Part model, mm, in its own coordinate system. A direction names the side the tool comes from. Coordinates: 2 decimals unless noted, no trailing zeros. Loops run counter-clockwise (first coordinate to the right, second up) from the corner with the lowest first, then second, coordinate; pieces in that order, holes last. Notation, with made-up numbers: (9.25, 62) -> (39.25, 62) arc R21 cw to (39.25, 100) -> close; hole circle Ø3 at (53.25, 4). An arc over 180 degrees is marked (long way). Use one line per item in the form item = value. Start each with the question number.
(1) Band-saw the part on C-C on z = 8. Give the cut face in (x, y), then the cut area to 3 significant figures.
(2) Band-saw the part on B-B on z = 38. Give the cut face in (x, y), then the cut area to 3 significant figures.
(3) 3-axis set-ups, long thin cutter, end or side, ignore diameter. For faces 1 (the flat face through (-30.894, -6.088, 0.493)), 2 (the flat face through (-6.35, 8, 6)), 3 (the flat face through (-30.37, -6.08, 24.66)): which of +Z, -Z, +X, -X, +Y, -Y reach the whole face in a straight line?
(4) Pin check, flat tips, straight feed: P1, Ø2, axis at x = -5, z = 21, coming from the -Y side; P2, Ø6, axis at y = 6, z = 42, coming from the +X side; P3, Ø1, axis at y = -5, z = 8, coming from the +X side. Stop position of each tip, or through.
(5) Band-saw the part on D-D on x = -3. Give the cut face in (y, z), then the cut area to 3 significant figures.
(6) Mould opens along Z. For faces 4 (the flat face through (-24, 3, 50)), 5 (the cylindrical face through (-3.131, 5.349, 46.957)), 6 (the flat face through (-34, -12, 25)) say: +Z half, -Z half, draft (parallel to the pull), parting line (faces both ways), or undercut.
(7) Band-saw the part on A-A on y = 6. Give the cut face in (x, z), then the cut area to 3 significant figures.
(8) Drill centre lines: L1, parallel to Z at x = -1.25, y = 6; L2, parallel to Z at x = -16, y = 6; L3, parallel to Y at x = -8, z = 12.5. Where is each one in solid material? Low to high. Write a range as [from, to].
```python
from build123d import *

# Parameters (mm, degrees)
F1_DEPTH       = 50
F3_D           = 5.1054
F3_CBORE_D     = 10
F3_CBORE_DEPTH = 6.35
F4_SIZE        = 1


with BuildPart() as f1:
    # F0 (on Top) → F1 (new body)
    with BuildSketch(Plane.XY):
        Polygon((-32, 0), (0, 0), (0, 12), (-38.78461, 12), (-38.78461, -12), (-28.78461, -12), align=None)
    extrude(amount=F1_DEPTH)

    # F3 (through all)
    with Locations(Plane.YZ):
        with Locations((6, 42), (6, 8)):
            CounterBoreHole(F3_D / 2, F3_CBORE_D / 2, F3_CBORE_DEPTH)

    # F4
    f4_edges = [f1.edges().sort_by_distance(p)[0] for p in [
        (-30.392305, -6, 50),
        (-30.392305, -6, 0),
    ]]
    chamfer(f4_edges, length=F4_SIZE)


solid = f1.part
```
A:
q1.outline = (-38.78, -12) -> (-28.78, -12) -> (-32, 0) -> (0, 0) -> (0, 1) -> (-6.35, 1) -> (-6.35, 3.45) -> (-38.78, 3.45) -> close; (-38.78, 8.55) -> (-6.35, 8.55) -> (-6.35, 11) -> (0, 11) -> (0, 12) -> (-38.78, 12) -> close
q1.area = 337 mm²
q2.outline = (-38.78, -12) -> (-28.78, -12) -> (-32, 0) -> (0, 0) -> (0, 3) -> (-6.35, 3) -> (-6.35, 9) -> (0, 9) -> (0, 12) -> (-38.78, 12) -> close
q2.area = 528 mm²
q3.face_1 = -Z, +X
q3.face_2 = +X
q3.face_3 = +Z, -Z, +X
q4.P1 = 0
q4.P2 = -6.35
q4.P3 = -30.53
q5.outline = (0, 0) -> (12, 0) -> (12, 50) -> (0, 50) -> close; hole circle Ø10 at (6, 8); hole circle Ø10 at (6, 42)
q5.area = 443 mm²
q6.face_4 = +Z half
q6.face_5 = undercut
q6.face_6 = draft
q7.outline = (-38.78, 0) -> (0, 0) -> (0, 3) -> (-6.35, 3) -> (-6.35, 5.45) -> (-38.78, 5.45) -> close; (-38.78, 10.55) -> (-6.35, 10.55) -> (-6.35, 13) -> (0, 13) -> (0, 37) -> (-6.35, 37) -> (-6.35, 39.45) -> (-38.78, 39.45) -> close; (-38.78, 44.55) -> (-6.35, 44.55) -> (-6.35, 47) -> (0, 47) -> (0, 50) -> (-38.78, 50) -> close
q7.area = 1,480 mm²
q8.L1 = [0, 3], [13, 37], [47, 50]
q8.L2 = [0, 5.45], [10.55, 39.45], [44.55, 50]
q8.L3 = [0, 12]
